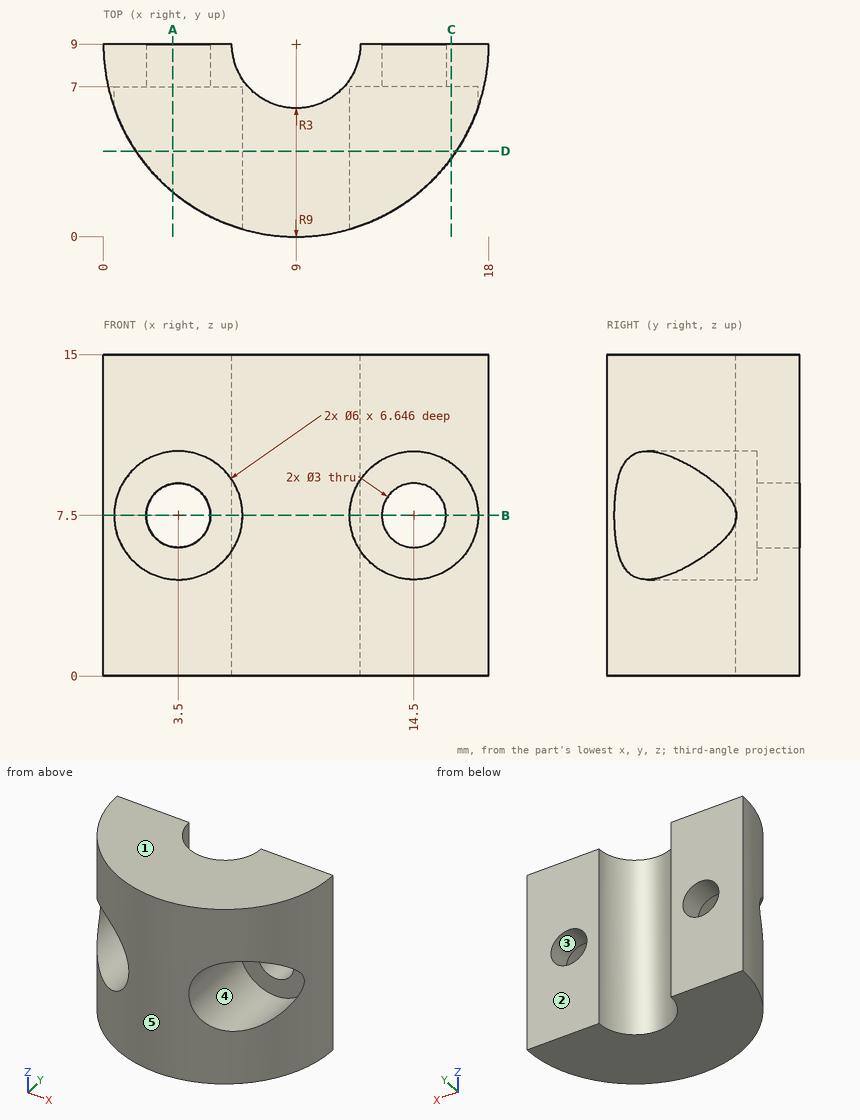
Check sheet for the drawn part. Datum: minimum x, y, z corner. Units: mm. A direction names the side the tool comes from. Give positions to 0.01 mm unless a question says otherwise; leave off trailing zeros. Order: outer loops, then holes, each group sorted by start corner. A loop starts at its lowest first (then second) coordinate and runs counter-clockwise, first axis right, second up.
1. Scan lines: line 1 (X direction, y = 7.55, z = 7.5); line 2 (X direction, y = 5.25, z = 7.5); line 3 (Y direction, x = 16.75, z = 8.5). Record each from-to range of solid material in increasing order.
Completed:
line 1: x = 0.12 to 2, 5 to 6.37, 11.63 to 13, 16 to 17.88
line 2: x = 6.5 to 11.5
line 3: y = 7 to 9
2. Draft check along Z on the marked faces 1, 2 and 3. Enter one of: pulls with the +Z half, pulls with the -Z half, needs draft (parallel to the pull), parting line crosses it, or undercut.
Completed:
face 1: pulls with the +Z half
face 2: needs draft
face 3: undercut
3. Sectioned sample at B-B (z = 7.5). Record the boundary of the cut face in (x, y).
Completed:
outline: (0, 9) arc R9 ccw to (0.5, 6.04) - (0.5, 7) - (2, 7) - (2, 9) - close; (5, 7) - (6.5, 7) - (6.5, 0.35) arc R9 ccw to (11.5, 0.35) - (11.5, 7) - (13, 7) - (13, 9) - (12, 9) arc R3 cw to (6, 9) - (5, 9) - close; (16, 7) - (17.5, 7) - (17.5, 6.04) arc R9 ccw to (18, 9) - (16, 9) - close
4. Access from +Z, -Z, +X, -X, +Y, -Y to the whole of each face (thin tool, end or side, straight path). Record for the marked faces 4 and 5.
Completed:
face 4: -Y
face 5: +Z, -Z, -Y
5. Depth check by flat-ended pin: pin 1 (4 mm diameter, centred on x = 3.5, z = 7.5, fed in from -Y); pin 2 (6.5 mm diameter, centred on x = 4, z = 8.5, fed in from -Y); pin 3 (8 mm diameter, centred on x = 13.5, z = 9, fed in from -Y). Enter the tip coordinate at first touch or a pass-through.
Completed:
pin 1: stops at y = 7
pin 2: stops at y = 0.17
pin 3: stops at y = 0.01
6. Sectioned sample at D-D (y = 4). Record the boundary of the cut face in (x, z).
Completed:
outline: (1.52, 0) - (16.48, 0) - (16.48, 5.25) arc R3 cw (long way) to (16.48, 9.75) - (16.48, 15) - (1.52, 15) - (1.52, 9.75) arc R3 cw (long way) to (1.52, 5.25) - close
7. Sectioned sample at C-C (x = 16.25). Record the boundary of the cut face in (y, z).
Completed:
outline: (3.67, 0) - (9, 0) - (9, 15) - (3.67, 15) - (3.67, 9.94) - (7, 9.94) - (7, 5.06) - (3.67, 5.06) - close
8. Sectioned sample at A-A (x = 3.25). Record the boundary of the cut face in (y, z).
Completed:
outline: (2.08, 0) - (9, 0) - (9, 6.02) - (7, 6.02) - (7, 4.51) - (2.08, 4.51) - close; (2.08, 10.49) - (7, 10.49) - (7, 8.98) - (9, 8.98) - (9, 15) - (2.08, 15) - close
